from build123d import *

# Parameters (mm, degrees)
SKETCH3_R           = 47.125
SKETCH3_R_2         = 4
SKETCH3_R_3         = 2
BOSS_EXTRUDE1_DEPTH = 6
CHAMFER1_SIZE       = 2.5
CHAMFER1_SIZE2      = 2


with BuildPart() as part:
    # Sketch3 → Boss-Extrude1 (new body)
    with BuildSketch(Plane(origin=(0, 0, 0), x_dir=(0, 1, 0), z_dir=(0, 0, 1))):
        with Locations(Location((0, 0, 0), (0, 0, 270))):
            Circle(SKETCH3_R)
        with Locations(Location((0, 0, 0), (0, 0, 270))):
            Circle(SKETCH3_R_2, mode=Mode.SUBTRACT)
        with Locations(Location((26, 0, 0), (0, 0, 270))):
            Circle(SKETCH3_R_3, mode=Mode.SUBTRACT)
        with Locations(Location((-13, -22.516660498, 0), (0, 0, 270))):
            Circle(SKETCH3_R_3, mode=Mode.SUBTRACT)
        with Locations(Location((-13, 22.516660498, 0), (0, 0, 270))):
            Circle(SKETCH3_R_3, mode=Mode.SUBTRACT)
    extrude(amount=BOSS_EXTRUDE1_DEPTH)

    # Chamfer1
    chamfer1_edges = [part.edges().sort_by_distance(p)[0] for p in [
        (20.516660498, -13, 6),
        (-24.516660498, -13, 6),
        (-2, 26, 6),
    ]]
    chamfer1_side = [part.faces().sort_by_distance(p)[0] for p in [
        (-45.792103717, 0, 6),
    ]]
    chamfer(chamfer1_edges, length=CHAMFER1_SIZE, length2=CHAMFER1_SIZE2, reference=chamfer1_side[0])


solid = part.part
Design review of the part built by this model. Coordinates are the model's own, in mm. Round coordinates to 2 decimals unless told otherwise and drop trailing zeros. Write each loop counter-clockwise with the first axis right and the second up, starting at its lowest first coordinate (ties: lowest second). Pieces come first, ordered by that corner, then holes. Notation, with made-up numbers: (-16, 37) - (6, 37) arc R12 ccw to (6, 44) - close; hole circle Ø4 at (-20.75, 11.5). An arc over 180 degrees is marked (long way). Use a Markdown table: item, result. Add a question column.
1. We need section B-B (y = 0). State the section outline as (x, z) points (3 decimals).
2. Clearance check with flat-ended pins moving along their axes: pin 1 (1.5 mm diameter, centred on x = -9, z = 5, fed in from +Y); pin 2 (1 mm diameter, centred on x = 34, z = 1.5, fed in from -Y); pin 3 (6.5 mm diameter, centred on x = -22.52, y = -13, fed in from +Z). State where each tip first meets the part, or that it passes through.
3. We need section D-D (y = -13). State the section outline as (x, z) points.
4. Mouldability with a two-part tool opening along Y and no side actions: class faces 1 (the face through (-1, -10, 0)), 2 (the face through (20.83, -14.29, 4.1)), 3 (the face through (44.949, 14.155, 2.958)) as +Y half, -Y half, draft (parallel to the pull), parting line (faces both ways), or undercut.
5. We need section A-A (x = 0). State the section outline as (y, z) points (3 decimals).
6. Wall thickness on probe 1 along Y at (x, z) = (0, 2.2) (3 decimals); probe 2 along Y at (x, z) = (-24, 5.7); probe 3 along X at (y, z) = (-24.5, 4.4): over which ranges is each line inside the solid? List them lowest first.
7. We need section C-C (z = 2). State the section outline as (x, y) points (3 decimals), then the cut area to 3 significant figures.
Output:
| question | item | result |
|---|---|---|
| 1 | outline | (-47.125, 0) - (-4, 0) - (-4, 6) - (-47.125, 6) - close; (4, 0) - (47.125, 0) - (47.125, 6) - (4, 6) - close |
| 2 | pin 1 | stops at y = 46.4 |
| 2 | pin 2 | stops at y = -33.14 |
| 2 | pin 3 | stops at z = 5 |
| 3 | outline | (-45.3, 0) - (-24.52, 0) - (-24.52, 4) - (-27.02, 6) - (-45.3, 6) - close; (-20.52, 0) - (20.52, 0) - (20.52, 4) - (18.02, 6) - (-18.02, 6) - (-20.52, 4) - close; (24.52, 0) - (45.3, 0) - (45.3, 6) - (27.02, 6) - (24.52, 4) - close |
| 4 | face 1 | draft |
| 4 | face 2 | undercut |
| 4 | face 3 | parting line |
| 5 | outline | (-47.125, 0) - (-4, 0) - (-4, 6) - (-47.125, 6) - close; (4, 0) - (24, 0) - (24, 4) - (21.5, 6) - (4, 6) - close; (28, 0) - (47.125, 0) - (47.125, 6) - (30.5, 6) - (28, 4) - close |
| 6 | probe 1 | y = -47.125 to -4, 4 to 24, 28 to 47.125 |
| 6 | probe 2 | y = -40.56 to -16.85, -9.15 to 40.56 |
| 6 | probe 3 | x = -40.26 to 40.26 |
| 7 | outline | circle Ø94.25 at (0, 0); hole circle Ø4 at (-22.517, -13); hole circle Ø8 at (0, 0); hole circle Ø4 at (0, 26); hole circle Ø4 at (22.517, -13) |
| 7 | area | 6,890 mm2 |
